Geometry: final body of the model. Coordinates: model frame, mm. Face numbers are marked on the shaded views. A direction names the side the tool comes from. Give positions to 0.01 mm unless a question says otherwise; leave off trailing zeros. Write each loop counter-clockwise with the first axis right and the second up, starting at its lowest first coordinate (ties: lowest second). Pieces come first, ordered by that corner, then holes.
Autodesk Inventor part; units mm, degrees
ref_plane "YZ Plane" through (0, 0, 0) normal (1, 0, 0) x (0, 1, 0)
ref_plane "XZ Plane" through (0, 0, 0) normal (0, 1, 0) x (-1, 0, 0)
ref_plane "XY Plane" through (0, 0, 0) normal (0, 0, 1) x (1, 0, 0)
sketch "Sketch1" plane through (0, 0, 0) normal (0, 0, 1) x (1, 0, 0)
  circle A0 centre (0, 0) radius 1.8
  circle A1 centre (0, 0) radius 17
  circle A2 centre (0, 0) radius 7.5
  circle A3 centre (0, 0) radius 24
  circle A4 centre (20.75, 0) radius 1.8
  circle A5 centre (14.6725, 14.6725) radius 1.8
  circle A6 centre (0, 20.75) radius 1.8
  circle A7 centre (-14.6725, 14.6725) radius 1.8
  circle A8 centre (-20.75, 0) radius 1.8
  circle A9 centre (-14.6725, -14.6725) radius 1.8
  circle A10 centre (0, -20.75) radius 1.8
  circle A11 centre (14.6725, -14.6725) radius 1.8
  dimension "d0" = 3.6
  dimension "d1" = 34
  dimension "d2" = 15
  dimension "d3" = 48
  dimension "d4" = 3.6
  dimension "d5" = 20.75
  dimension "d8" = 360
extrude "Extrusion1" add sketch "Sketch1" along normal blind 2 contours A1 | A2 | A3
extrude "Extrusion2" add sketch "Sketch1" along normal blind 10 contours A3
fillet "Fillet1" radius 2 1 edges at (-17, 0, 2)
extrude "Extrusion3" add sketch "Sketch1" along normal blind 18 contours A2
properties part number "MoldeB"
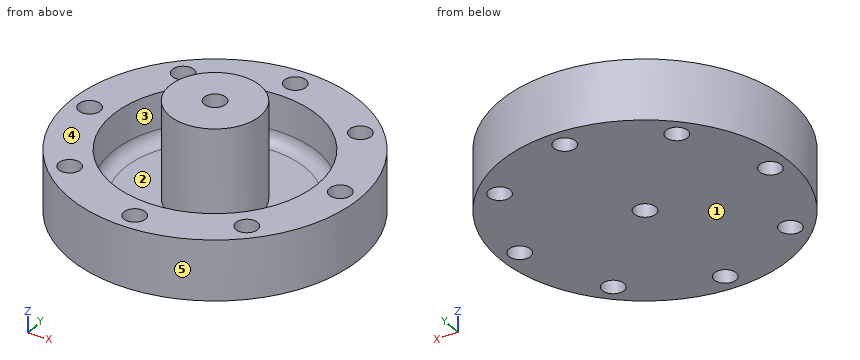
Item 1: Section C-C, the plane z = 9.25. State how many separate pieces and enclosed holes the cut face has, plus the area to 3 significant figures.
Found:
separate pieces: 2
enclosed holes: 10
area: 987 mm2
Item 2: Pin query (flat end, axial travel): pin 1 Ø1.5 at (x, z) = (1, 12) entering from -Y; pin 2 Ø6 at (y, z) = (-8, 3.5) entering from +X; pin 3 Ø6 at (x, y) = (20.75, 0) entering from +Z. Return the tip coordinate at first contact, or that it passes through.
Found:
pin 1: stops at y = -7.5
pin 2: stops at x = 23.47
pin 3: stops at z = 10
Item 3: Reachability of the marked faces 1 and 2 from +Z, -Z, +X, -X, +Y, -Y: full face, straight path, thin tool, end or side. Return the list, or none.
Found:
face 1: -Z, +X, -X, +Y, -Y
face 2: +Z
Item 4: Section A-A, the plane x = 0. Return the cut outline in (y, z), plus the area to 3 significant figures.
Found:
outline: (-24, 0) - (-22.55, 0) - (-22.55, 10) - (-24, 10) - close; (-18.95, 0) - (-1.8, 0) - (-1.8, 18) - (-7.5, 18) - (-7.5, 2) - (-15, 2) arc R2 cw to (-17, 4) - (-17, 10) - (-18.95, 10) - close; (1.8, 0) - (18.95, 0) - (18.95, 10) - (17, 10) - (17, 4) arc R2 cw to (15, 2) - (7.5, 2) - (7.5, 18) - (1.8, 18) - close; (22.55, 0) - (24, 0) - (24, 10) - (22.55, 10) - close
area: 313 mm2
Item 5: Pull-direction query (Y, two-part tool) for the marked faces 3, 4 and 5; classes: +Y half, -Y half, draft (parallel to the pull), parting line (faces both ways), or undercut.
Found:
face 3: undercut
face 4: draft
face 5: parting line
Item 6: Section D-D, the plane x = 20.75. Return the cut outline in (y, z), plus the area to 3 significant figures.
Found:
outline: (-12.06, 0) - (-1.8, 0) - (-1.8, 10) - (-12.06, 10) - close; (1.8, 0) - (12.06, 0) - (12.06, 10) - (1.8, 10) - close
area: 205 mm2
Item 7: Line query: L1, parallel to Y at x = 0, z = 5.25; L2, parallel to X at y = 5.5, z = 4.25; L3, parallel to X at y = -6, z = 4.25. Output: solid intervals per line, ascending.
Found:
L1: y = -24 to -22.55, -18.95 to -17, -7.5 to -1.8, 1.8 to 7.5, 17 to 18.95, 22.55 to 24
L2: x = -23.36 to -16.09, -5.1 to 5.1, 16.09 to 23.36
L3: x = -23.24 to -15.91, -4.5 to 4.5, 15.91 to 23.24
